Source: CAD feature listing. Evaluate the final solid. Frame: model axes, mm. A direction names the side the tool comes from. Give positions to 0.01 mm unless a question says otherwise; leave off trailing zeros. Order: outer loops, then holes, each group sorted by start corner. A loop starts at its lowest first (then second) coordinate and runs counter-clockwise, first axis right, second up. Notation, with made-up numbers: M 46.25,71 L 89.25,71 A19 ccw 89.25,78 Z; hole C -14.5,77.25 d10. An arc over 180 degrees is marked long. Answer in a Markdown table with one row per item. Add a question column.
(1) Set-up query: faces 5 (the face through (29.235, 96.027, 14.234)), 6 (the face through (25.01, 101.24, 12)). Return all of +Z, -Z, +X, -X, +Y, -Y with unobstructed straight access to the full face (end or side cutting, diameter ignored); none if empty.
(2) Pin query (flat end, axial travel): P1, Ø7, axis at x = 15.74, y = 99.69, coming from the -Z side; P2, Ø6, axis at x = 16, y = 128, coming from the -Z side; P3, Ø2.5, axis at x = 17, y = 100, coming from the -Z side. Return the tip coordinate at first contact, or that it passes through.
(3) Section query A-A, the plane x = 15.25. Return loops of the section in (y, z).
(4) Section query D-D, the plane x = 20.5. Return loops of the section in (y, z).
(5) Material intervals for line 1 along X through (y, z) = (99, 11); line 2 along Y through (x, z) = (12.5, 12.5); line 3 along Y through (x, z) = (19.25, 11.75), sorted ascending.
(6) Mould query, pull axis X, two halves, no side actions, for faces 1 (the face through (24, 129, 12)), 2 (the face through (14.55, 98.78, 13.23)), 3 (the face through (11.7, 109.09, 1.33)), 4 (the face through (29.7, 119.98, 1.35)). Classes: pulls with the +X half, pulls with the -X half, needs draft (parallel to the pull), parting line crosses it, or undercut.
(7) Section query B-B, the plane y = 130.5. Return loops of the section in (x, z).
(8) Section query C-C, the plane z = 8. Return loops of the section in (x, y).
from build123d import *

# Parameters (mm, degrees)
SKETCH2_W           = 20
SKETCH2_H           = 49.6
SKETCH2_R           = 1.5
BOSS_EXTRUDE1_DEPTH = 30
CUT_EXTRUDE1_DEPTH  = 30
CUT_EXTRUDE2_DEPTH  = 22
FILLET1_R           = 5
FILLET2_R           = 2
CHAMFER1_SIZE       = 2
SKETCH5_R           = 3
SKETCH5_R_2         = 1.5
CUT_EXTRUDE3_DEPTH  = 12
CUT_EXTRUDE4_DEPTH  = 23


with BuildPart() as part:
    # Sketch2 → Boss-Extrude1 (new body)
    with BuildSketch(Plane.XY):
        with Locations((20.689228864, 114.541105708)):
            Rectangle(SKETCH2_W, SKETCH2_H)
        with Locations((15.739481395, 99.69135824)):
            Circle(SKETCH2_R, mode=Mode.SUBTRACT)
        with Locations((25.638976332, 99.69135824)):
            Circle(SKETCH2_R, mode=Mode.SUBTRACT)
        with Locations((25.638976332, 129.390853177)):
            Circle(SKETCH2_R, mode=Mode.SUBTRACT)
        with Locations((15.739481395, 129.390853177)):
            Circle(SKETCH2_R, mode=Mode.SUBTRACT)
    extrude(amount=BOSS_EXTRUDE1_DEPTH)

    # Sketch3 → Cut-Extrude1 (cut)
    with BuildSketch(Plane(origin=(30.689228864, 0, 0), x_dir=(0, 0, -1), z_dir=(1, 0, 0))):
        Polygon((-10, 119.541105708), (-18.024193548, 119.541105708), (-11.975806452, 109.541105708), (-10, 109.541105708), align=None)
        Polygon((-11.975806452, 109.541105708), (-18.024193548, 119.541105708), (-20, 119.541105708), (-20, 109.541105708), align=None)
    extrude(amount=-CUT_EXTRUDE1_DEPTH, mode=Mode.SUBTRACT)

    # Sketch4 → Cut-Extrude2 (cut)
    with BuildSketch(Plane(origin=(30.689228864, 0, 0), x_dir=(0, 0, -1), z_dir=(1, 0, 0))):
        Polygon((-30, 139.341105708), (-27.096774194, 134.541105708), (-15, 134.541105708), (0, 134.541105708), (0, 139.341105708), align=None)
        Polygon((-30, 134.541105708), (-27.096774194, 134.541105708), (-30, 139.341105708), align=None)
        Polygon((-15, 134.541105708), (0, 120.541105708), (0, 134.541105708), align=None)
        Polygon((-7.268041237, 101.757600554), (-2.903225806, 94.541105708), (0, 94.541105708), (0, 108.541105708), align=None)
        Polygon((-15, 94.541105708), (-2.903225806, 94.541105708), (-7.268041237, 101.757600554), align=None)
        Polygon((-30, 89.741105708), (0, 89.741105708), (-2.903225806, 94.541105708), (-15, 94.541105708), (-30, 94.541105708), align=None)
        Polygon((-2.903225806, 94.541105708), (0, 89.741105708), (0, 94.541105708), align=None)
    extrude(amount=-CUT_EXTRUDE2_DEPTH, mode=Mode.SUBTRACT)

    # Fillet1
    fillet1_edges = [part.edges().sort_by_distance(p)[0] for p in [
        (20.689228864, 134.541105708, 15),
        (20.689228864, 120.541105708, 0),
        (20.689228864, 94.541105708, 15),
        (20.689228864, 108.541105708, 0),
    ]]
    fillet(fillet1_edges, radius=FILLET1_R)

    # Fillet2
    fillet2_edges = [part.edges().sort_by_distance(p)[0] for p in [
        (20.689228864, 134.541105708, 30),
        (20.689228864, 94.541105708, 30),
    ]]
    fillet(fillet2_edges, radius=FILLET2_R)

    # Chamfer1
    chamfer1_edges = [part.edges().sort_by_distance(p)[0] for p in [
        (30.689228864, 127.610001295, 7.5738167),
        (10.689228864, 127.610001295, 7.5738167),
        (30.689228864, 114.541105708, 0),
        (30.689228864, 101.472210122, 7.5738167),
        (30.689228864, 108.721124919, 0.414263622),
        (30.689228864, 120.361086498, 0.414263622),
        (30.689228864, 94.889418826, 15.137292206),
        (30.689228864, 134.192792591, 15.137292206),
        (10.689228864, 114.541105708, 0),
        (10.689228864, 101.472210122, 7.5738167),
        (10.689228864, 108.721124919, 0.414263622),
        (10.689228864, 120.361086498, 0.414263622),
        (10.689228864, 94.889418826, 15.137292206),
        (10.689228864, 134.192792591, 15.137292206),
        (10.689228864, 114.541105708, 30),
        (30.689228864, 114.541105708, 30),
        (30.689228864, 134.541105708, 22.485407952),
        (30.689228864, 94.541105708, 22.485407952),
        (30.689228864, 133.955319271, 29.414213562),
        (30.689228864, 95.126892146, 29.414213562),
        (10.689228864, 94.541105708, 22.485407952),
        (10.689228864, 134.541105708, 22.485407952),
        (10.689228864, 133.955319271, 29.414213562),
        (10.689228864, 95.126892146, 29.414213562),
    ]]
    chamfer(chamfer1_edges, length=CHAMFER1_SIZE - 0.0001)  # a hair under: the kernel refuses the full size

    # Sketch5 → Cut-Extrude3 (cut)
    # profile 1 of 4: a face of its own
    with BuildSketch(Plane(origin=(0, 0, 0), x_dir=(-1, 0, 0), z_dir=(0, 0, -1))):
        with Locations((-15.739481395, 99.69135824)):
            Circle(SKETCH5_R)
        with Locations((-15.739481395, 99.69135824)):
            Circle(SKETCH5_R_2, mode=Mode.SUBTRACT)
    # profile 2 of 4: a face of its own
    with BuildSketch(Plane(origin=(0, 0, 0), x_dir=(-1, 0, 0), z_dir=(0, 0, -1))):
        with Locations((-25.638976332, 99.69135824)):
            Circle(SKETCH5_R)
        with Locations((-25.638976332, 99.69135824)):
            Circle(SKETCH5_R_2, mode=Mode.SUBTRACT)
    # profile 3 of 4: a face of its own
    with BuildSketch(Plane(origin=(0, 0, 0), x_dir=(-1, 0, 0), z_dir=(0, 0, -1))):
        with Locations((-15.739481395, 129.390853177)):
            Circle(SKETCH5_R)
        with Locations((-15.739481395, 129.390853177)):
            Circle(SKETCH5_R_2, mode=Mode.SUBTRACT)
    # profile 4 of 4: a face of its own
    with BuildSketch(Plane(origin=(0, 0, 0), x_dir=(-1, 0, 0), z_dir=(0, 0, -1))):
        with Locations((-25.638976332, 129.390853177)):
            Circle(SKETCH5_R)
        with Locations((-25.638976332, 129.390853177)):
            Circle(SKETCH5_R_2, mode=Mode.SUBTRACT)
    extrude(amount=-CUT_EXTRUDE3_DEPTH, mode=Mode.SUBTRACT)

    # Sketch6 → Cut-Extrude4 (cut)
    with BuildSketch(Plane.ZY.offset(-10.689228864)):
        with BuildLine():
            ThreePointArc((16.970815903, 96.541105708), (16.478743483, 96.581736733), (16, 96.70252922))
            Line((16, 96.70252922), (16, 91.202832585))
            Line((16, 91.202832585), (39.910531439, 91.202832585))
            Line((39.910531439, 91.202832585), (39.910531439, 137.879378832))
            Line((39.910531439, 137.879378832), (16, 137.879378832))
            Line((16, 137.879378832), (16, 132.379682197))
            ThreePointArc((16, 132.379682197), (16.478743483, 132.500474684), (16.970815903, 132.541105708))
            Line((16.970815903, 132.541105708), (28, 132.541105708))
            Line((28, 132.541105708), (28, 96.541105708))
            Line((28, 96.541105708), (16.970815903, 96.541105708))
        make_face()
        with BuildLine():
            ThreePointArc((23, 114.541105708), (21, 109.249603086), (16, 106.603851775))
            Line((16, 106.603851775), (16, 96.70252922))
            ThreePointArc((16, 96.70252922), (16.478743483, 96.581736733), (16.970815903, 96.541105708))
            Line((16.970815903, 96.541105708), (28, 96.541105708))
            Line((28, 96.541105708), (28, 132.541105708))
            Line((28, 132.541105708), (16.970815903, 132.541105708))
            ThreePointArc((16.970815903, 132.541105708), (16.478743483, 132.500474684), (16, 132.379682197))
            Line((16, 132.379682197), (16, 122.478359641))
            ThreePointArc((16, 122.478359641), (21, 119.83260833), (23, 114.541105708))
        make_face()
        Polygon((20, 119.541105708), (16, 115.541105708), (16, 109.541105708), (20, 109.541105708), align=None)
        Polygon((16, 119.541105708), (16, 115.541105708), (20, 119.541105708), align=None)
        with BuildLine():
            Line((14.5, 109.541105708), (10, 109.541105708))
            Line((10, 109.541105708), (10, 119.541105708))
            Line((10, 119.541105708), (14.5, 119.541105708))
            Line((14.5, 119.541105708), (14.5, 122.52546542))
            ThreePointArc((14.5, 122.52546542), (7, 114.541105708), (14.5, 106.556745997))
            Line((14.5, 106.556745997), (14.5, 109.541105708))
        make_face()
        with BuildLine():
            Line((20, 109.541105708), (16, 109.541105708))
            Line((16, 109.541105708), (16, 106.603851775))
            ThreePointArc((16, 106.603851775), (21, 109.249603086), (23, 114.541105708))
            ThreePointArc((23, 114.541105708), (21, 119.83260833), (16, 122.478359641))
            Line((16, 122.478359641), (16, 119.541105708))
            Line((16, 119.541105708), (20, 119.541105708))
            Line((20, 119.541105708), (20, 109.541105708))
        make_face()
        Polygon((10, 119.541105708), (10, 109.541105708), (14.5, 114.041105708), (14.5, 119.541105708), align=None)
        with BuildLine():
            Line((14.5, 122.52546542), (14.5, 119.541105708))
            Line((14.5, 119.541105708), (15, 119.541105708))
            Line((15, 119.541105708), (15, 122.541105708))
            ThreePointArc((15, 122.541105708), (14.749877721, 122.53719468), (14.5, 122.52546542))
        make_face()
        with BuildLine():
            Line((15, 122.541105708), (15, 119.541105708))
            Line((15, 119.541105708), (16, 119.541105708))
            Line((16, 119.541105708), (16, 122.478359641))
            ThreePointArc((16, 122.478359641), (15.5009833, 122.525403782), (15, 122.541105708))
        make_face()
        Polygon((14.5, 119.541105708), (14.5, 114.041105708), (15, 114.541105708), (15, 119.541105708), align=None)
        Polygon((15, 119.541105708), (15, 114.541105708), (16, 115.541105708), (16, 119.541105708), align=None)
        Polygon((14.5, 114.041105708), (10, 109.541105708), (14.5, 109.541105708), align=None)
        Polygon((15, 114.541105708), (14.5, 114.041105708), (14.5, 109.541105708), (15, 109.541105708), align=None)
        Polygon((16, 115.541105708), (15, 114.541105708), (15, 109.541105708), (16, 109.541105708), align=None)
        with BuildLine():
            Line((15, 109.541105708), (14.5, 109.541105708))
            Line((14.5, 109.541105708), (14.5, 106.556745997))
            ThreePointArc((14.5, 106.556745997), (14.749877721, 106.545016736), (15, 106.541105708))
            Line((15, 106.541105708), (15, 109.541105708))
        make_face()
        with BuildLine():
            Line((16, 109.541105708), (15, 109.541105708))
            Line((15, 109.541105708), (15, 106.541105708))
            ThreePointArc((15, 106.541105708), (15.5009833, 106.556807634), (16, 106.603851775))
            Line((16, 106.603851775), (16, 109.541105708))
        make_face()
        with BuildLine():
            ThreePointArc((15, 106.541105708), (14.749877721, 106.545016736), (14.5, 106.556745997))
            Line((14.5, 106.556745997), (14.5, 97.743543645))
            Line((14.5, 97.743543645), (14.923861152, 97.347939904))
            ThreePointArc((14.923861152, 97.347939904), (14.961637209, 97.313281439), (15, 97.279273558))
            Line((15, 97.279273558), (15, 106.541105708))
        make_face()
        with BuildLine():
            ThreePointArc((16, 106.603851775), (15.5009833, 106.556807634), (15, 106.541105708))
            Line((15, 106.541105708), (15, 97.279273558))
            ThreePointArc((15, 97.279273558), (15.471997059, 96.942347914), (16, 96.70252922))
            Line((16, 96.70252922), (16, 106.603851775))
        make_face()
        with BuildLine():
            Line((14.923861152, 97.347939904), (14.5, 97.743543645))
            Line((14.5, 97.743543645), (14.5, 91.202832585))
            Line((14.5, 91.202832585), (15, 91.202832585))
            Line((15, 91.202832585), (15, 97.279273558))
            ThreePointArc((15, 97.279273558), (14.961637209, 97.313281439), (14.923861152, 97.347939904))
        make_face()
        with BuildLine():
            ThreePointArc((16, 96.70252922), (15.471997059, 96.942347914), (15, 97.279273558))
            Line((15, 97.279273558), (15, 91.202832585))
            Line((15, 91.202832585), (16, 91.202832585))
            Line((16, 91.202832585), (16, 96.70252922))
        make_face()
        with BuildLine():
            Line((14.5, 131.338667771), (14.5, 122.52546542))
            ThreePointArc((14.5, 122.52546542), (14.749877721, 122.53719468), (15, 122.541105708))
            Line((15, 122.541105708), (15, 131.802937859))
            ThreePointArc((15, 131.802937859), (14.961637209, 131.768929978), (14.923861152, 131.734271513))
            Line((14.923861152, 131.734271513), (14.5, 131.338667771))
        make_face()
        with BuildLine():
            Line((15, 131.802937859), (15, 122.541105708))
            ThreePointArc((15, 122.541105708), (15.5009833, 122.525403782), (16, 122.478359641))
            Line((16, 122.478359641), (16, 132.379682197))
            ThreePointArc((16, 132.379682197), (15.471997059, 132.139863502), (15, 131.802937859))
        make_face()
        with BuildLine():
            Line((14.5, 137.879378832), (14.5, 131.338667771))
            Line((14.5, 131.338667771), (14.923861152, 131.734271513))
            ThreePointArc((14.923861152, 131.734271513), (14.961637209, 131.768929978), (15, 131.802937859))
            Line((15, 131.802937859), (15, 137.879378832))
            Line((15, 137.879378832), (14.5, 137.879378832))
        make_face()
        with BuildLine():
            Line((15, 137.879378832), (15, 131.802937859))
            ThreePointArc((15, 131.802937859), (15.471997059, 132.139863502), (16, 132.379682197))
            Line((16, 132.379682197), (16, 137.879378832))
            Line((16, 137.879378832), (15, 137.879378832))
        make_face()
    extrude(amount=-CUT_EXTRUDE4_DEPTH, mode=Mode.SUBTRACT)


solid = part.part
Values follow:
| question | item | result |
|---|---|---|
| 1 | face 5 | -Z, +X, -Y |
| 1 | face 6 | -Z |
| 2 | P1 | stops at z = 5.73 |
| 2 | P2 | stops at z = 4.78 |
| 2 | P3 | stops at z = 12 |
| 3 | outline | M 95.19,14.5 A5 ccw 95.89,13.56 L 97.34,12 L 98.27,12 L 98.27,14.5 Z; M 101.11,12 L 102.65,12 L 102.65,6.31 L 107.06,1.59 A5 ccw 110.71,0 L 118.37,0 A5 ccw 122.02,1.59 L 126.43,6.31 L 126.43,12 L 127.97,12 L 127.97,14.5 L 122.53,14.5 A8 cw 106.56,14.5 L 101.11,14.5 Z; M 130.81,12 L 131.74,12 L 133.2,13.56 A5 ccw 133.89,14.5 L 130.81,14.5 Z |
| 4 | outline | M 95.19,14.5 A5 ccw 95.89,13.56 L 107.06,1.59 A5 ccw 110.71,0 L 118.37,0 A5 ccw 122.02,1.59 L 133.2,13.56 A5 ccw 133.89,14.5 L 122.53,14.5 A8 cw 106.56,14.5 Z |
| 5 | line 1 | x = 12.16 to 12.82, 18.66 to 22.72, 28.56 to 29.22 |
| 5 | line 2 | y = 97.13 to 106.94, 122.14 to 131.95 |
| 5 | line 3 | y = 97.57 to 107.23, 121.85 to 131.51 |
| 6 | face 1 | undercut |
| 6 | face 2 | undercut |
| 6 | face 3 | pulls with the -X half |
| 6 | face 4 | pulls with the +X half |
| 7 | outline | M 10.69,13.6 L 12.69,10.67 L 12.95,10.67 L 12.95,12 L 14.73,12 L 14.73,14.5 L 10.69,14.5 Z; M 16.75,12 L 18.53,12 L 18.53,10.67 L 22.85,10.67 L 22.85,12 L 24.63,12 L 24.63,14.5 L 16.75,14.5 Z; M 26.65,12 L 28.43,12 L 28.43,10.67 L 28.69,10.67 L 30.69,13.6 L 30.69,14.5 L 26.65,14.5 Z |
| 8 | outline | M 10.69,103.81 L 12.69,101.07 L 13.08,101.07 A3 cw 18.4,101.07 L 22.98,101.07 A3 cw 28.3,101.07 L 28.69,101.07 L 30.69,103.81 L 30.69,110.67 L 10.69,110.67 Z; M 10.69,118.41 L 30.69,118.41 L 30.69,125.27 L 28.69,128.01 L 28.3,128.01 A3 cw 22.98,128.01 L 18.4,128.01 A3 cw 13.08,128.01 L 12.69,128.01 L 10.69,125.27 Z |
